Autodesk Inventor part; units mm, degrees
ref_plane "YZ Plane" through (0, 0, 0) normal (1, 0, 0) x (0, 1, 0)
ref_plane "XZ Plane" through (0, 0, 0) normal (0, 1, 0) x (-1, 0, 0)
ref_plane "XY Plane" through (0, 0, 0) normal (0, 0, 1) x (1, 0, 0)
sketch "Sketch1" plane through (0, 0, 0) normal (0, 1, 0) x (-1, 0, 0)
  circle A0 centre (0, 0) radius 1
  line L0 (2, 2) -> (-2, 2)
  line L1 (-2, 2) -> (-2, -12.16)
  line L2 (-2, -12.16) -> (2, -12.16)
  line L3 (2, -12.16) -> (2, 2)
  circle A1 centre (0, -2.54) radius 1
  circle A2 centre (0, -5.08) radius 1
  circle A3 centre (0, -7.62) radius 1
  circle A4 centre (0, -10.16) radius 1
  dimension "d0" = 2
  dimension "d3" = 2.54
  dimension "d8" = 1
  dimension "d9" = 1
  dimension "d10" = 1
  dimension "d11" = 1
extrude "Extrusion1" add sketch "Sketch1" along normal blind 10.5
equation "\"d9\" = d8"
equation "\"d10\" = d8"
equation "\"d11\" = d8"
properties part number "Encoder Header Spacer 2"
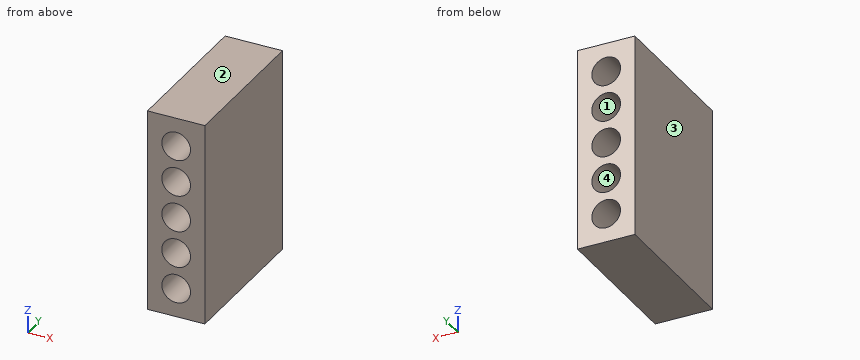
Could you check a few things on this model? Use its own coordinates, in mm. Face numbers are marked on the shaded views. Give positions to 0.01 mm unless a question says otherwise; leave off trailing zeros. Loops run counter-clockwise (first coordinate to the right, second up) from the corner with the lowest first, then second, coordinate; pieces in that order, holes last. Notation, with made-up numbers: M -15.75,52.5 L 23.25,52.5 A35 cw 23.25,88.5 Z; hole C -28,72.5 d11. An arc over 180 degrees is marked long. Answer as a JSON object with one key per item and string values.
Q1. Suppose I cut it at C-C, the plane y = 1. List the corners of the cut face in (x, z) for me, plus the area to 3 significant figures.
Values found:
{"outline": "M -2,-12.16 L 2,-12.16 L 2,2 L -2,2 Z; hole C 0,-10.16 d2; hole C 0,-7.62 d2; hole C 0,-5.08 d2; hole C 0,-2.54 d2; hole C 0,0 d2", "area": "40.9 mm²"}
Q2. If I drill on probe 1 along Z at (x, y) = (0, 7.25); probe 2 along Z at (x, y) = (-0.6, 5); probe 3 along X at (y, z) = (2.75, -0.25), over which ranges is the centre line in solid material (lowest first)? Write a range as [from, to].
Values found:
{"probe 1": "z = [-12.16, -11.16], [-9.16, -8.62], [-6.62, -6.08], [-4.08, -3.54], [-1.54, -1], [1, 2]", "probe 2": "z = [-12.16, -10.96], [-9.36, -8.42], [-6.82, -5.88], [-4.28, -3.34], [-1.74, -0.8], [0.8, 2]", "probe 3": "x = [-2, -0.97], [0.97, 2]"}
Q3. If we mould it in two halves opening along Z, with no side actions, what happens to the marked faces 1, 2, 3 and 4? For each: pulls with the +Z half, pulls with the -Z half, needs draft (parallel to the pull), parting line crosses it, or undercut.
Values found:
{"face 1": "undercut", "face 2": "pulls with the +Z half", "face 3": "needs draft", "face 4": "undercut"}
Q4. Suppose I cut it at A-A, the plane x = -0.8. List the corners of the cut face in (y, z) for me, plus the area to 3 significant figures.
Values found:
{"outline": "M 0,-12.16 L 10.5,-12.16 L 10.5,-10.76 L 0,-10.76 Z; M 0,-9.56 L 10.5,-9.56 L 10.5,-8.22 L 0,-8.22 Z; M 0,-7.02 L 10.5,-7.02 L 10.5,-5.68 L 0,-5.68 Z; M 0,-4.48 L 10.5,-4.48 L 10.5,-3.14 L 0,-3.14 Z; M 0,-1.94 L 10.5,-1.94 L 10.5,-0.6 L 0,-0.6 Z; M 0,0.6 L 10.5,0.6 L 10.5,2 L 0,2 Z", "area": "85.7 mm²"}
Q5. Suppose I cut it at B-B, the plane z = 0. List the corners of the cut face in (x, y) for me.
Values found:
{"outline": "M -2,0 L -1,0 L -1,10.5 L -2,10.5 Z; M 1,0 L 2,0 L 2,10.5 L 1,10.5 Z"}
Q6. Suppose I cut it at D-D, the plane x = 0. List the corners of the cut face in (y, z) for me.
Values found:
{"outline": "M 0,-12.16 L 10.5,-12.16 L 10.5,-11.16 L 0,-11.16 Z; M 0,-9.16 L 10.5,-9.16 L 10.5,-8.62 L 0,-8.62 Z; M 0,-6.62 L 10.5,-6.62 L 10.5,-6.08 L 0,-6.08 Z; M 0,-4.08 L 10.5,-4.08 L 10.5,-3.54 L 0,-3.54 Z; M 0,-1.54 L 10.5,-1.54 L 10.5,-1 L 0,-1 Z; M 0,1 L 10.5,1 L 10.5,2 L 0,2 Z"}
Q7. For P1, Ø1.8, axis at x = 0, z = 0, coming from the -Y side, with a flat end and sliding along its axis, tell me the tip position at first contact or that it passes through.
Values found:
{"P1": "passes through"}
